Autodesk Inventor part; units mm, degrees
ref_plane "Work Plane1" through (27.9676, -72.374, -408.43) normal (-1, 0, 0) x (0, 0, 1)
ref_plane "YZ Plane" through (0, 0, 0) normal (1, 0, 0) x (0, 1, 0)
ref_plane "XZ Plane" through (0, 0, 0) normal (0, 1, 0) x (-1, 0, 0)
sketch "Sketch1" plane through (0, 0, 0) normal (0, 0, 1) x (1, 0, 0)
  line L0 (-4.826, 0.413) -> (-4.826, -0.413)
  line L1 (-2.826, -2.413) -> (4.826, -2.413)
  line L2 (4.826, -2.413) -> (4.826, 2.413)
  line L3 (4.826, 2.413) -> (-2.826, 2.413)
  arc A0 (-4.826, -0.413) -> (-2.826, -2.413) centre (-2.826, -0.413) ccw
  arc A1 (-2.826, 2.413) -> (-4.826, 0.413) centre (-2.826, 0.413) ccw
  point P0 (0, 0)
extrude "Extrusion1" add sketch "Sketch1" along normal blind 10
sketch "Sketch2" plane through (4.826, -2.413, 0) normal (1, 0, 0) x (0, 0, -1)
  line L0 (0, 0) -> (-10, 0)
  line L1 (-10, 0) -> (-10, 4.826)
  circle A0 centre (3.175, 150.3292) radius 1.5
  circle A1 centre (3.175, 23.749) radius 1.5
  circle A2 centre (73.025, 23.749) radius 1.5
  circle A3 centre (73.025, 150.3292) radius 1.5
  arc A4 (60.2046, 236.2874) -> (0.9041, 211.5001) centre (77.9391, 110.5317) ccw
  ellipse E0 centre (170.686, 87.0391) end of major axis (408.43, 87.0391) minor radius 177.8 (0.9041, 211.5001) -> (0.9041, -37.4219) ccw
  arc A5 (0.9041, -37.4219) -> (60.2046, -62.2092) centre (77.9391, 63.5465) ccw
  arc A6 (60.2046, -62.2092) -> (281.1673, -62.2092) centre (170.686, 721.2179) ccw
  arc A7 (281.1673, -62.2092) -> (340.4678, -37.4219) centre (263.4329, 63.5465) ccw
  ellipse E1 centre (170.686, 87.0391) end of major axis (408.43, 87.0391) minor radius 177.8 (340.4678, -37.4219) -> (340.4678, 211.5001) ccw
  arc A8 (340.4678, 211.5001) -> (281.1673, 236.2874) centre (263.4329, 110.5317) ccw
  arc A9 (281.1673, 236.2874) -> (60.2046, 236.2874) centre (170.686, -547.1397) ccw
  circle A10 centre (18.1159, 118.5546) radius 1.25
  circle A11 centre (-51.7341, 53.7756) radius 1.25
  circle A12 centre (18.1159, 53.7756) radius 1.25
  circle A13 centre (-51.7341, 118.5546) radius 1.25
  circle A14 centre (395.605, 77.7641) radius 1.25
  circle A15 centre (321.1037, 62.7821) radius 1.25
  circle A16 centre (321.1037, 101.1361) radius 1.25
  circle A17 centre (395.605, 96.3141) radius 1.25
  line L2 (284.5488, 72.0792) -> (223.628, 72.0792)
  line L3 (223.628, 72.0792) -> (223.628, 102.5592)
  line L4 (223.628, 102.5592) -> (284.5488, 102.5592)
  line L5 (284.5488, 102.5592) -> (284.5488, 72.0792)
  circle A18 centre (129.4087, 87.0391) radius 30.4
  line L6 (95.6616, 45.3432) -> (95.6616, 49.3432)
  arc A19 (98.6614, 49.3432) -> (95.6616, 49.3432) centre (97.1615, 49.3432) ccw
  line L7 (98.6614, 49.3432) -> (98.6614, 45.3432)
  arc A20 (95.6616, 45.3432) -> (98.6614, 45.3432) centre (97.1615, 45.3432) ccw
  line L8 (160.3503, 45.3892) -> (160.3503, 49.3892)
  arc A21 (163.3501, 49.3892) -> (160.3503, 49.3892) centre (161.8502, 49.3892) ccw
  line L9 (163.3501, 49.3892) -> (163.3501, 45.3892)
  arc A22 (160.3503, 45.3892) -> (163.3501, 45.3892) centre (161.8502, 45.3892) ccw
  line L10 (95.5803, 159.8921) -> (95.5803, 163.8921)
  arc A23 (98.5801, 163.8921) -> (95.5803, 163.8921) centre (97.0802, 163.8921) ccw
  line L11 (98.5801, 163.8921) -> (98.5801, 159.8921)
  arc A24 (95.5803, 159.8921) -> (98.5801, 159.8921) centre (97.0802, 159.8921) ccw
  line L12 (163.3504, 163.8921) -> (163.3504, 159.8921)
  arc A25 (160.3506, 159.8921) -> (163.3504, 159.8921) centre (161.8505, 159.8921) ccw
  line L13 (160.3506, 159.8921) -> (160.3506, 163.8921)
  arc A26 (163.3504, 163.8921) -> (160.3506, 163.8921) centre (161.8505, 163.8921) ccw
  arc A27 (180.3755, 134.9774) -> (180.3753, 131.9798) centre (180.3755, 133.4786) ccw
  line L14 (180.3755, 134.9774) -> (184.3754, 134.9776)
  arc A28 (184.3754, 131.9796) -> (184.3754, 134.9776) centre (184.3755, 133.4786) ccw
  line L15 (184.3754, 131.9796) -> (180.3753, 131.9798)
  arc A29 (65.9852, 134.9725) -> (65.9851, 131.9749) centre (65.9852, 133.4737) ccw
  line L16 (65.9852, 134.9725) -> (69.9852, 134.9727)
  arc A30 (69.9852, 131.9747) -> (69.9852, 134.9727) centre (69.9852, 133.4737) ccw
  line L17 (69.9852, 131.9747) -> (65.9851, 131.9749)
  arc A31 (188.0254, 134.9778) -> (188.0255, 131.9802) centre (188.0255, 133.479) ccw
  line L18 (188.0254, 134.9778) -> (192.0254, 134.978)
  arc A32 (192.0254, 131.98) -> (192.0254, 134.978) centre (192.0255, 133.479) ccw
  line L19 (192.0254, 131.98) -> (188.0255, 131.9802)
  arc A33 (73.6382, 70.1265) -> (73.6381, 67.1289) centre (73.6382, 68.6277) ccw
  line L20 (73.6382, 70.1265) -> (77.6381, 70.1267)
  arc A34 (77.6381, 67.1287) -> (77.6381, 70.1267) centre (77.6382, 68.6277) ccw
  line L21 (77.6381, 67.1287) -> (73.6381, 67.1289)
  circle A35 centre (271.4412, 59.8872) radius 1.25
  circle A36 centre (229.978, 118.4342) radius 1.25
  circle A37 centre (281.3738, 108.9092) radius 1.25
  circle A38 centre (278.1988, 118.4342) radius 1.25
  circle A39 centre (254.0826, 118.4342) radius 1.25
  circle A40 centre (226.803, 108.9092) radius 1.25
  circle A41 centre (226.5872, 59.8872) radius 1.25
  arc A42 (188.0714, 70.2078) -> (188.0714, 67.2102) centre (188.0714, 68.709) ccw
  line L22 (188.0714, 70.2078) -> (192.0714, 70.208)
  arc A43 (192.0714, 67.21) -> (192.0714, 70.208) centre (192.0714, 68.709) ccw
  line L23 (192.0714, 67.21) -> (188.0714, 67.2102)
  line L24 (73.6352, 134.9725) -> (77.6351, 134.9727)
  arc A44 (77.6351, 131.9747) -> (77.6351, 134.9727) centre (77.6352, 133.4737) ccw
  line L25 (77.6351, 131.9747) -> (73.6351, 131.9749)
  arc A45 (73.6352, 134.9725) -> (73.6351, 131.9749) centre (73.6352, 133.4737) ccw
  arc A46 (66.0312, 70.1211) -> (66.0311, 67.1235) centre (66.0312, 68.6223) ccw
  line L26 (66.0312, 70.1211) -> (70.0312, 70.1213)
  arc A47 (70.0312, 67.1233) -> (70.0312, 70.1213) centre (70.0312, 68.6223) ccw
  line L27 (70.0312, 67.1233) -> (66.0311, 67.1235)
  arc A48 (180.4215, 70.2024) -> (180.4213, 67.2048) centre (180.4215, 68.7036) ccw
  line L28 (180.4215, 70.2024) -> (184.4214, 70.2025)
  arc A49 (184.4214, 67.2046) -> (184.4214, 70.2025) centre (184.4215, 68.7036) ccw
  line L29 (184.4214, 67.2046) -> (180.4213, 67.2048)
  line L30 (160.3503, 152.2421) -> (160.3503, 156.2421)
  arc A50 (163.3501, 156.2421) -> (160.3503, 156.2421) centre (161.8502, 156.2421) ccw
  line L31 (163.3501, 156.2421) -> (163.3501, 152.2421)
  arc A51 (160.3503, 152.2421) -> (163.3501, 152.2421) centre (161.8502, 152.2421) ccw
  line L32 (95.5857, 152.1961) -> (95.5857, 156.1961)
  arc A52 (98.5855, 156.1961) -> (95.5857, 156.1961) centre (97.0856, 156.1961) ccw
  line L33 (98.5855, 156.1961) -> (98.5855, 152.1961)
  arc A53 (95.5857, 152.1961) -> (98.5855, 152.1961) centre (97.0856, 152.1961) ccw
  line L34 (160.3503, 37.7392) -> (160.3503, 41.7392)
  arc A54 (163.3501, 41.7392) -> (160.3503, 41.7392) centre (161.8502, 41.7392) ccw
  line L35 (163.3501, 41.7392) -> (163.3501, 37.7392)
  arc A55 (160.3503, 37.7392) -> (163.3501, 37.7392) centre (161.8502, 37.7392) ccw
  line L36 (95.667, 37.6932) -> (95.667, 41.6932)
  arc A56 (98.6669, 41.6932) -> (95.667, 41.6932) centre (97.167, 41.6932) ccw
  line L37 (98.6669, 41.6932) -> (98.6669, 37.6932)
  arc A57 (95.667, 37.6932) -> (98.6669, 37.6932) centre (97.167, 37.6932) ccw
  line L38 (0, 4.826) -> (-10, 4.826)
  line L39 (0, -10.668) -> (0, 15.494)
  circle A58 centre (-5, -5.334) radius 1.5
  circle A59 centre (81.2, -5.334) radius 1.5
  circle A60 centre (81.2, 10.16) radius 1.5
  circle A61 centre (-5, 10.16) radius 1.5
  circle A62 centre (-5, 163.9182) radius 1.5
  circle A63 centre (81.2, 163.9182) radius 1.5
  circle A64 centre (81.2, 179.4122) radius 1.5
  circle A65 centre (-5, 179.4122) radius 1.5
  circle A66 centre (73.025, 187.9212) radius 1.5
  circle A67 centre (73.025, -13.843) radius 1.5
  circle A68 centre (3.175, -13.843) radius 1.5
  circle A69 centre (3.175, 187.9212) radius 1.5
  circle A70 centre (268.3469, 187.9212) radius 1.5
  circle A71 centre (260.1719, 179.4122) radius 1.5
  circle A72 centre (346.3719, 10.16) radius 1.5
  circle A73 centre (346.3719, -5.334) radius 1.5
  circle A74 centre (346.3719, 179.4122) radius 1.5
  circle A75 centre (338.1969, 150.3292) radius 1.5
  circle A76 centre (260.1719, -5.334) radius 1.5
  circle A77 centre (268.3469, 23.749) radius 1.5
  circle A78 centre (268.3469, -13.843) radius 1.5
  circle A79 centre (260.1719, 10.16) radius 1.5
  circle A80 centre (268.3469, 150.3292) radius 1.5
  circle A81 centre (338.1969, -13.843) radius 1.5
  circle A82 centre (338.1969, 23.749) radius 1.5
  circle A83 centre (260.1719, 163.9182) radius 1.5
  circle A84 centre (338.1969, 187.9212) radius 1.5
  circle A85 centre (346.3719, 163.9182) radius 1.25
  point P0 (0, 2.413)
ref_plane "Work Plane1" through (27.9676, -72.374, -408.43) normal (-1, 0, 0) x (0, 0, 1)
extrude "Extrusion2" add sketch "Sketch2" along normal up to surface (23.1416 mm away) contours L0 L1 L38 L39
sketch "Sketch3" plane through (27.9676, -2.413, 10) normal (1, 0, 0) x (0, 0, -1)
  line L0 (10, -10.668) -> (10, 15.494)
  line L1 (10, -10.668) -> (0, -10.668)
  line L2 (0, -10.668) -> (0, 15.494)
  line L3 (0, 15.494) -> (10, 15.494)
  line L4 (10, 15.494) -> (10, -10.668)
  line L5 (10, 2.826) -> (10, 2)
  line L6 (10, 0) -> (10, -10.668)
  line L7 (10, 4.826) -> (10, 15.494)
  circle A0 centre (5, -5.334) radius 1.25
  circle A1 centre (5, 10.16) radius 1.25
  point P0 (10, 2.413)
  point P1 (5, -10.668)
  point P2 (5, 15.494)
  point P3 (10, -5.334)
  point P4 (10, 10.16)
  dimension "d4" = 2.5
  dimension "d5" = 2.5
extrude "Extrusion3" add sketch "Sketch3" against normal blind 2
sketch "Sketch4" plane through (0, 0, 0) normal (0, 0, -1) x (-1, 0, 0)
  circle A0 centre (-4.174, 0) radius 2.3
  line L0 (-4.174, 2.3) -> (-4.174, 2.413)
  line L1 (2.826, 2.413) -> (-25.9676, 2.413)
  line L2 (-4.174, -2.3) -> (-4.174, -2.413)
  line L3 (2.826, -2.413) -> (-25.9676, -2.413)
  line L4 (-25.9676, 2.413) -> (-25.9676, -2.413)
  line L5 (-4.174, -2.413) -> (-4.174, 2.413)
  line L6 (2.826, -2.413) -> (-25.9676, -2.413)
  arc A1 (4.826, -0.413) -> (2.826, -2.413) centre (2.826, -0.413) ccw
  line L7 (4.826, 0.413) -> (4.826, -0.413)
  arc A2 (2.826, 2.413) -> (4.826, 0.413) centre (2.826, 0.413) ccw
  line L8 (2.826, 2.413) -> (-25.9676, 2.413)
  line L9 (-27.9676, 13.081) -> (-25.9676, 13.081)
  line L10 (-27.9676, -13.081) -> (-27.9676, 13.081)
  line L11 (-27.9676, -13.081) -> (-25.9676, -13.081)
  line L12 (-25.9676, -2.413) -> (-25.9676, -13.081)
  line L13 (-4.174, 2.413) -> (11.7475, 2.413)
  line L14 (11.7475, 2.413) -> (11.7475, -2.413)
  line L15 (11.7475, -2.413) -> (-4.174, -2.413)
  point P0 (0, 0)
extrude "Extrusion4" cut sketch "Sketch4" against normal blind 10 contours A0 L5 | A0 L0 L1 A2 A1 L3 L2 | A2 L7 A1 | A1 A2 | L13 L14 L15 A1 A2 picked at (-3.8414, 0.6907)
sketch "Sketch5" plane through (0, 0, 0) normal (0, 0, -1) x (-1, 0, 0)
  circle A0 centre (-4.174, 0) radius 2.413
  point P0 (0, 0)
extrude "Extrusion5" add sketch "Sketch5" against normal blind 10
fillet "Fillet2" radius 1 1 edges at (1.761, 0, 10)
fillet "Fillet3" radius 1 4 edges at (26.9676, 13.081, 10) (26.9676, 13.081, 0) (26.9676, -13.081, 10) (26.9676, -13.081, 0)
properties part number "GuideArmConnector"
Input: part model. Units: mm. Frame: model coordinates. A direction names the side the tool comes from. Give positions to 0.01 mm unless a question says otherwise; leave off trailing zeros. Order: outer loops, then holes, each group sorted by start corner. A loop starts at its lowest first (then second) coordinate and runs counter-clockwise, first axis right, second up. Notation, with made-up numbers: (81, -6) -> (92, -6) arc R25 ccw to (92, 11) -> close; hole circle Ø8 at (21, 56.5). An arc over 180 degrees is marked (long way). Write each question's results on one line, items separated by ' | '. Start each with the question number.
Item 1: Set-up query: faces 4 (the cylindrical face through (14.918, -2.128, 9.699)), 5 (the cylindrical face through (15.223, 2.128, 9.699)), 6 (the flat face through (15, 2.413, 4)). Return all of +Z, -Z, +X, -X, +Y, -Y with unobstructed straight access to the full face (end or side cutting, diameter ignored); none if empty.
Item 2: Cut plane D-D on y = 4.25. Return the cut outline in (x, z).
Item 3: Cut plane A-A on z = 5. Return the cut outline in (x, y), then the cut area to 3 significant figures.
Item 4: Contact query for flat-ended pins moving along their axis: P1, Ø6, axis at x = 16.5, z = 8.5, coming from the -Y side; P2, Ø2.5, axis at x = 11, z = 2.5, coming from the +Y side. Output: stop coordinate, or through.
Item 5: Line query: line 1 (Y direction, x = 26.4, z = 5); line 2 (X direction, y = 4, z = 4); line 3 (Y direction, x = 10, z = 5.75). Output: solid intervals per line, ascending.
Item 6: Mould query, pull axis Z, two halves, no side actions, for faces 1 (the cylindrical face through (26.954, -12.796, 9.699)), 2 (the cylindrical face through (26.982, -8.967, 5.271)), 3 (the cylindrical face through (26.954, 12.796, 0.301)). Classes: pulls with the +Z half, pulls with the -Z half, needs draft (parallel to the pull), parting line crosses it, or undercut.
Item 7: Cut plane B-B on z = 1.5. Return the cut outline in (x, y), then the cut area to 3 significant figures.
Item 8: Cut plane C-C on x = 21. Return the cut outline in (y, z).
Established:
1) face 4: +Z, -X, -Y | face 5: +Z, -X, +Y | face 6: +Z, -Z, -X, +Y
2) outline: (25.97, 0) -> (27.97, 0) -> (27.97, 10) -> (25.97, 10) -> close
3) outline: (4.17, -2.41) -> (25.97, -2.41) -> (25.97, -6.5) -> (27.97, -6.5) -> (27.97, 6.5) -> (25.97, 6.5) -> (25.97, 2.41) -> (4.17, 2.41) arc R2.41 ccw to start; (25.97, -13.08) -> (27.97, -13.08) -> (27.97, -9) -> (25.97, -9) -> close; (25.97, 9) -> (27.97, 9) -> (27.97, 13.08) -> (25.97, 13.08) -> close | area: 157 mm^2
4) P1: y = -2.41 | P2: y = 2.41
5) line 1: -13.08 to -9, -6.5 to 6.5, 9 to 13.08 | line 2: 25.97 to 27.97 | line 3: -2.41 to 2.41
6) face 1: pulls with the +Z half | face 2: undercut | face 3: pulls with the -Z half
7) outline: (4.17, -2.41) -> (25.97, -2.41) -> (25.97, -13.08) -> (27.97, -13.08) -> (27.97, 13.08) -> (25.97, 13.08) -> (25.97, 2.41) -> (4.17, 2.41) arc R2.41 ccw to start | area: 167 mm^2
8) outline: (-2.41, 0) -> (2.41, 0) -> (2.41, 9) arc R1 ccw to (1.41, 10) -> (-1.41, 10) arc R1 ccw to (-2.41, 9) -> close
